from build123d import *

# Parameters (mm, degrees)
SKETCH_1_W      = 20
SKETCH_1_H      = 3
EXTRUDE_1_DEPTH = 1.5


with BuildPart() as part:
    # 草图1 → 凸台-拉伸1 (new body, symmetric)
    with BuildSketch(Plane.XY):
        Polygon((-25, 20), (25, 20), (25, 10), (22, 10), (22, 2), (19, 2), (19, 5.265909841), (16, 5.265909841), (16, 2), (15, 2), (15, -2), (16, -2), (16, -5.769694942), (19, -5.769694942), (19, -2), (22, -2), (22, -10), (25, -10), (25, -20), (-25, -20), align=None)
        with Locations((0, -16.5)):
            Rectangle(SKETCH_1_W, SKETCH_1_H, mode=Mode.SUBTRACT)
    extrude(amount=EXTRUDE_1_DEPTH, both=True)


solid = part.part
CAD build for the part. Positions are in the model's coordinates, mm. A direction names the side the tool comes from. Coordinates: 2 decimals unless noted, no trailing zeros. Write each loop counter-clockwise with the first axis right and the second up, starting at its lowest first coordinate (ties: lowest second). Pieces come first, ordered by that corner, then holes. Notation, with made-up numbers: M 19.25,55.25 L 43.25,55.25 A10 ccw 43.25,70.25 Z; hole C 41.5,3.5 d10. An arc over 180 degrees is marked long. Answer as a JSON object with one key per item and string values. Group by question number.
1) Wall check: line 1 (Y direction, x = -9.5, z = 0.3); line 2 (X direction, y = -6.5, z = 0.9); line 3 (X direction, y = -16, z = -0.9). Give the ranges that are in metal, low to high. Write a range as from..to.
2) Saw through at D-D (y = -0.5). Write the cut outline in (x, z), plus the area to 3 significant figures.
3) Saw through at C-C (z = -1). Write the cut outline in (x, y).
4) Mould opens along X. For faces 4 (the face through (0, -20, 0)), 5 (the face through (25, -15, 0)), 6 (the face through (16, 4, 0)) say: +X half, -X half, draft (parallel to the pull), parting line (faces both ways), or undercut.
5) Saw through at A-A (y = -17). Write the cut outline in (x, z).
6) Saw through at B-B (x = -8). Write the cut outline in (y, z).
7) Pin check, flat tips, straight feed: pin 1 Ø0.9 at (y, z) = (6.5, 0.5) entering from +X; pin 2 Ø0.9 at (y, z) = (0.5, 0) entering from +X. Stop position of each tip, or through.
8) Tool access for faces 1 (the face through (17, -5.77, 0)), 2 (the face through (0, 0, 1.5)), 3 (the face through (20, -2, 0)): list every direction of +Z, -Z, +X, -X, +Y, -Y with a clear straight run to the whole face (end or side of a thin tool).
Values follow:
{
 "1": {"line 1": "y = -20..-18, -15..20", "line 2": "x = -25..22", "line 3": "x = -25..-10, 10..25"},
 "2": {"outline": "M -25,-1.5 L 15,-1.5 L 15,1.5 L -25,1.5 Z", "area": "120 mm2"},
 "3": {"outline": "M -25,-20 L 25,-20 L 25,-10 L 22,-10 L 22,-2 L 19,-2 L 19,-5.77 L 16,-5.77 L 16,-2 L 15,-2 L 15,2 L 16,2 L 16,5.27 L 19,5.27 L 19,2 L 22,2 L 22,10 L 25,10 L 25,20 L -25,20 Z; hole M -10,-18 L 10,-18 L 10,-15 L -10,-15 Z"},
 "4": {"face 4": "draft", "face 5": "+X half", "face 6": "undercut"},
 "5": {"outline": "M -25,-1.5 L -10,-1.5 L -10,1.5 L -25,1.5 Z; M 10,-1.5 L 25,-1.5 L 25,1.5 L 10,1.5 Z"},
 "6": {"outline": "M -20,-1.5 L -18,-1.5 L -18,1.5 L -20,1.5 Z; M -15,-1.5 L 20,-1.5 L 20,1.5 L -15,1.5 Z"},
 "7": {"pin 1": "stops at x = 22", "pin 2": "stops at x = 15"},
 "8": {"face 1": "+Z, -Z", "face 2": "+Z, +X, -X, +Y, -Y", "face 3": "+Z, -Z, +X"}
}
